from build123d import *

# Parameters (mm, degrees)
SKETCH_W        = 31
SKETCH_H        = 31
PAD_DEPTH       = 11
SKETCH001_W     = 25.5
SKETCH001_H     = 25.5
POCKET_DEPTH    = 7
SKETCH002_W     = 6
SKETCH002_H     = 9
POCKET001_DEPTH = 2
SKETCH003_R     = 1.5
POCKET002_DEPTH = 5
SKETCH004_W     = 7.912528
SKETCH004_H     = 3
POCKET003_DEPTH = 5


with BuildPart() as part:
    # Sketch → Pad (new body)
    with BuildSketch(Plane.XY):
        with Locations((15.5, 15.5)):
            Rectangle(SKETCH_W, SKETCH_H)
    extrude(amount=PAD_DEPTH)

    # Sketch001 (on Face6 of Pad) → Pocket (cut)
    with BuildSketch(Plane.XY.offset(11)):
        with Locations((15.5, 15.5)):
            Rectangle(SKETCH001_W, SKETCH001_H)
    extrude(amount=-POCKET_DEPTH, mode=Mode.SUBTRACT)

    # Sketch002 (on Face11 of Pocket) → Pocket001 (cut)
    with BuildSketch(Plane.XY.offset(4)):
        with Locations((7, 22.5)):
            Rectangle(SKETCH002_W, SKETCH002_H)
    extrude(amount=-POCKET001_DEPTH, mode=Mode.SUBTRACT)

    # Sketch003 (on Face16 of Pocket001) → Pocket002 (cut)
    with BuildSketch(Plane.XY.offset(2)):
        with Locations((7, 25)):
            Circle(SKETCH003_R)
        with Locations((7, 20)):
            Circle(SKETCH003_R)
    extrude(amount=-POCKET002_DEPTH, mode=Mode.SUBTRACT)

    # Sketch004 (on Face12 of Pocket002) → Pocket003 (cut)
    with BuildSketch(Plane.XZ.offset(-28.25)):
        with Locations((15.5, 5.5)):
            Rectangle(SKETCH004_W, SKETCH004_H)
    extrude(amount=-POCKET003_DEPTH, mode=Mode.SUBTRACT)


solid = part.part
The listing builds one solid part. Answer for the finished solid, in the listing's coordinates (mm). A direction names the side the tool comes from. Round coordinates to 2 decimals unless told otherwise and drop trailing zeros. Loops run counter-clockwise (first coordinate to the right, second up) from the corner with the lowest first, then second, coordinate; pieces in that order, holes last. Notation, with made-up numbers: M 71.5,65.25 L 129.5,65.25 A16 cw 129.5,75.25 Z; hole C 55.25,84.25 d8. An arc over 180 degrees is marked long. Return JSON: item names as keys, results as strings.
Q1. Which of the six approach directions +Z, -Z, +X, -X, +Y, -Y give full straight-line access (tool end or side, diameter ignored) to faces 1 (the face through (5.89, 21.01, 1.01)), 2 (the face through (11.544, 30, 5)), 3 (the face through (7, 27, 3))?
Results list:
{"face 1": "+Z, -Z", "face 2": "+Y", "face 3": "+Z"}
Q2. Find the intervals of material crossed by line 1 along Y through (x, z) = (7, 1.25); line 2 along Y through (x, z) = (3, 4.5); line 3 along X through (y, z) = (19, 3.75), in increasing order. Write a range as from..to.
Results list:
{"line 1": "y = 0..18.5, 21.5..23.5, 26.5..31", "line 2": "y = 0..2.75, 28.25..31", "line 3": "x = 0..4, 10..31"}
Q3. Find section D-D, the plane y = 9. Determine the outline of the cut face in (x, z), plus the area to 4 significant figures.
Results list:
{"outline": "M 0,0 L 31,0 L 31,11 L 28.25,11 L 28.25,4 L 2.75,4 L 2.75,11 L 0,11 Z", "area": "162.5 mm2"}
Q4. Find section B-B, the plane x = 7. Determine the outline of the cut face in (y, z), plus the area to 4 significant figures.
Results list:
{"outline": "M 0,0 L 18.5,0 L 18.5,2 L 18,2 L 18,4 L 2.75,4 L 2.75,11 L 0,11 Z; M 21.5,0 L 23.5,0 L 23.5,2 L 21.5,2 Z; M 26.5,0 L 31,0 L 31,11 L 28.25,11 L 28.25,4 L 27,4 L 27,2 L 26.5,2 Z", "area": "132.5 mm2"}
Q5. Find section A-A, the plane y = 20. Determine the outline of the cut face in (x, z), plus the area to 4 significant figures.
Results list:
{"outline": "M 0,0 L 5.5,0 L 5.5,2 L 4,2 L 4,4 L 2.75,4 L 2.75,11 L 0,11 Z; M 8.5,0 L 31,0 L 31,11 L 28.25,11 L 28.25,4 L 10,4 L 10,2 L 8.5,2 Z", "area": "144.5 mm2"}
Q6. Find section C-C, the plane z = 8.5. Determine the outline of the cut face in (x, y), plus the area to 3 significant figures.
Results list:
{"outline": "M 0,0 L 31,0 L 31,31 L 0,31 Z; hole M 2.75,2.75 L 28.25,2.75 L 28.25,28.25 L 2.75,28.25 Z", "area": "311 mm2"}
Q7. Each of these flat-tipped pins is pushed along its axis until it touches: pin 1 Ø2 at (y, z) = (30, 6) entering from -X; pin 2 Ø6.5 at (x, y) = (7, 23) entering from +Z. Where does it stop, or does it pass through?
Results list:
{"pin 1": "stops at x = 0", "pin 2": "stops at z = 4"}
Q8. The mould has two halves that part along Z. Classify faces 4 (the face through (15, 30, 7)), 5 (the face through (15, 16, 0)), 6 (the face through (19.456, 30, 5)), 7 (the face through (7, 18, 3)): released by +Z, released by -Z, zero draft, split by the parting line, or undercut.
Results list:
{"face 4": "undercut", "face 5": "released by -Z", "face 6": "undercut", "face 7": "zero draft"}
